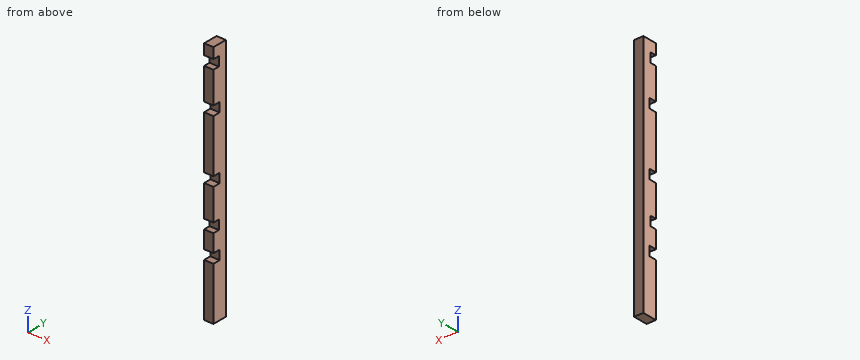
from build123d import *

# Parameters (mm, degrees)
F0_W     = 44
F0_H     = 69
F1_DEPTH = 1100
F2_W     = 30
F2_H     = 44
F3_DEPTH = 44.001
F4_W     = 34.5
F4_H     = 44
F5_DEPTH = 44.001
F6_DEPTH = 50
F7_W     = 34.5
F7_H     = 44
F8_DEPTH = 133


with BuildPart() as f1:
    # F0 (on Top) → F1 (new body)
    with BuildSketch(Plane.XY):
        Rectangle(F0_W, F0_H)
    extrude(amount=F1_DEPTH)

    # F2 (on face) → F3 (cut, through all)
    with BuildSketch(Plane.YZ.offset(22)):
        with Locations((-19.5, 1028)):
            Rectangle(F2_W, F2_H)
        with Locations((-19.5, 349)):
            Rectangle(F2_W, F2_H)
    extrude(amount=-F3_DEPTH, mode=Mode.SUBTRACT)

    # F4 (on face) → F5 (cut, through all)
    with BuildSketch(Plane.YZ.offset(22)):
        with Locations((-17.25, 835.5)):
            Rectangle(F4_W, F4_H)
        with Locations((-17.25, 541.5)):
            Rectangle(F4_W, F4_H)
    extrude(amount=-F5_DEPTH, mode=Mode.SUBTRACT)

    # F6 (add): a face of the model
    f6_faces = [f1.faces().sort_by_distance(p)[0] for p in [
        (0, 0, 0),
    ]]
    extrude(f6_faces, amount=F6_DEPTH)

    # F7 (on face) → F8 (cut)
    with BuildSketch(Plane.YZ.offset(22)):
        with Locations((-17.25, 222)):
            Rectangle(F7_W, F7_H)
    extrude(amount=-F8_DEPTH, mode=Mode.SUBTRACT)


solid = f1.part
Check sheet for the modelled part. Datum: model origin and axes. Units: mm. Give positions to 0.01 mm unless a question says otherwise; leave off trailing zeros. Loops run counter-clockwise (first coordinate to the right, second up) from the corner with the lowest first, then second, coordinate; pieces in that order, holes last. Notation, with made-up numbers: M 81,-10 L 129,-10 A31 ccw 129,23 Z; hole C 88.5,-29.75 d3. An arc over 180 degrees is marked long. Answer as a JSON object with one key per item and string values. Group by question number.
Q1. Go/stop test with flat-tipped pins: P1, Ø13, axis at x = -6.5, z = 345, coming from the -Y side; P2, Ø5, axis at x = 10.5, z = 844, coming from the -Y side. Record where each tip stops, or that it passes through.
Q2. Material ranges on line 1 along Z through (x, y) = (6, -8); line 2 along Z through (x, y) = (-5, -3.5); line 3 along Y through (x, z) = (-16, 1043), recorded low to high. Write a range as [from, to].
Q3. Cross-section at A-A on x = -4. Record the cut outline in (y, z).
Evaluation:
{
 "1": {"P1": "stops at y = -4.5", "P2": "stops at y = 0"},
 "2": {"line 1": "z = [-50, 200], [244, 327], [371, 519.5], [563.5, 813.5], [857.5, 1006], [1050, 1100]", "line 2": "z = [-50, 200], [244, 519.5], [563.5, 813.5], [857.5, 1100]", "line 3": "y = [-4.5, 34.5]"},
 "3": {"outline": "M -34.5,-50 L 34.5,-50 L 34.5,1100 L -34.5,1100 L -34.5,1050 L -4.5,1050 L -4.5,1006 L -34.5,1006 L -34.5,857.5 L 0,857.5 L 0,813.5 L -34.5,813.5 L -34.5,563.5 L 0,563.5 L 0,519.5 L -34.5,519.5 L -34.5,371 L -4.5,371 L -4.5,327 L -34.5,327 L -34.5,244 L 0,244 L 0,200 L -34.5,200 Z"}
}
